Autodesk Inventor part; units mm, degrees
ref_plane "YZ Plane" through (0, 0, 0) normal (1, 0, 0) x (0, 1, 0)
ref_plane "XZ Plane" through (0, 0, 0) normal (0, 1, 0) x (-1, 0, 0)
ref_plane "XY Plane" through (0, 0, 0) normal (0, 0, 1) x (1, 0, 0)
sketch "Sketch1" plane through (0, 0, 0) normal (0, 0, 1) x (1, 0, 0)
  circle A0 centre (0, 0) radius 11.7
  dimension "d0" = 23.4
extrude "Extrusion1" add sketch "Sketch1" along normal blind 15
sketch "Sketch2" plane through (0, 0, 0) normal (0, 0, -1) x (-1, 0, 0)
  circle A0 centre (0, 0) radius 11.7
  line L0 (-11.7, 0) -> (-11.7, -20)
  line L1 (-11.7, -20) -> (11.7, -20)
  line L2 (11.7, -20) -> (11.7, 0)
  circle A1 centre (0, 0) radius 11.7
  line L3 (-11.7, 0) -> (11.7, 0)
  point P0 (11.7, 0)
  point P1 (-11.7, 0)
  dimension "d3" = 20
extrude "Extrusion2" add sketch "Sketch2" along normal blind 10
sketch "Sketch3" plane through (-11.7, -20, 0) normal (0, -1, 0) x (1, 0, 0)
  line L0 (-4.3, 22) -> (27.7, 22)
  line L1 (27.7, 22) -> (27.7, -10)
  line L2 (27.7, -10) -> (-4.3, -10)
  line L3 (-4.3, -10) -> (-4.3, 22)
  line L4 (23.4, -10) -> (0, -10)
  line L5 (23.4, 0) -> (0, 0)
  point P0 (11.7, 0)
  point P1 (11.7, 22)
  point P2 (11.7, 0)
  dimension "d6" = 32
  dimension "d7" = 32
extrude "Extrusion3" add sketch "Sketch3" along normal blind 10
sketch "Sketch4" plane through (-11.7, -30, 0) normal (0, -1, 0) x (1, 0, 0)
  line L0 (0.7, 17) -> (22.7, 17) construction
  line L1 (22.7, 17) -> (22.7, -5) construction
  line L2 (22.7, -5) -> (0.7, -5) construction
  line L3 (0.7, -5) -> (0.7, 17) construction
  line L4 (27.7, 22) -> (-4.3, 22) construction
  line L5 (-4.3, 22) -> (-4.3, -10) construction
  point P0 (11.7, 0)
  point P1 (11.7, 17)
  point P2 (11.7, 22)
  point P3 (0.7, 6)
  point P4 (-4.3, 6)
  dimension "d10" = 22
  dimension "d11" = 22
hole "Hole1" at (-11, -30, 17) at (11, -30, 17) at (11, -30, -5) at (-11, -30, -5) direction (0, 1, 0) diameter 5 depth 10
sketch "Sketch5" plane through (0, 0, 0) normal (0, 0, 1) x (1, 0, 0)
  line L0 (11.7, -20) -> (-11.7, -20)
  line L1 (5, -20) -> (-5, -20)
  line L2 (-5, -20) -> (-5, -11.7)
  line L3 (-5, -11.7) -> (5, -11.7)
  line L4 (5, -11.7) -> (5, -20)
  circle A0 centre (0, 0) radius 11.7
  line L5 (11.7, -20) -> (5, -20)
  line L6 (5, -20) -> (5, -14)
  line L7 (5, -14) -> (11.7, -14)
  line L8 (11.7, -14) -> (11.7, -20)
  line L9 (-5, -20) -> (-11.7, -20)
  line L10 (-11.7, -20) -> (-11.7, -14)
  line L11 (-11.7, -14) -> (-5, -14)
  line L12 (-5, -14) -> (-5, -20)
  line L13 (-11.7, -20) -> (-11.7, 0)
  line L14 (11.7, 0) -> (11.7, -20)
  point P0 (0, -11.7)
  dimension "d19" = 10
  dimension "d20" = 6
extrude "Extrusion4" cut sketch "Sketch5" against normal through all contours L0 L4 L7 L8 | L0 L10 L11 L2
chamfer "Chamfer1" distance 1 distance2 3 1 edges at (-11.7, 0, 15) measured on face at (-1.2696, -2.7132, 15)
equation "\"d7\" = d6"
equation "\"d11\" = d10"
properties part number "0008-30-004"
Source: CAD feature listing. Evaluate the final solid. Frame: model axes, mm. A direction names the side the tool comes from. Give positions to 0.01 mm unless a question says otherwise; leave off trailing zeros. Order: outer loops, then holes, each group sorted by start corner. A loop starts at its lowest first (then second) coordinate and runs counter-clockwise, first axis right, second up. Notation, with made-up numbers: (37.25, 59) -> (42.25, 59) arc R29 ccw to (42.25, 96) -> close; hole circle Ø1 at (67.25, 19). An arc over 180 degrees is marked (long way). Write item = value, one per line.
Item 1: Mould query, pull axis Y, two halves, no side actions, for faces 5 (the face through (5.4, 10.38, 3.29)), 6 (the face through (11.7, -7, -5)), 7 (the face through (0, -30, 6)). Classes: +Y half, -Y half, draft (parallel to the pull), parting line (faces both ways), or undercut.
Check result:
face_5 = undercut
face_6 = draft
face_7 = -Y half
Item 2: Section query A-A (z = -5). Output: boundary loops of the cut face in (x, y), then the cut area to 3 significant figures.
Check result:
outline = (-16, -30) -> (-13.5, -30) -> (-13.5, -20) -> (-16, -20) -> close; (-11.7, -14) -> (-5, -14) -> (-5, -20) -> (-8.5, -20) -> (-8.5, -30) -> (8.5, -30) -> (8.5, -20) -> (5, -20) -> (5, -14) -> (11.7, -14) -> (11.7, 0) arc R11.7 ccw to (-11.7, 0) -> close; (13.5, -30) -> (16, -30) -> (16, -20) -> (13.5, -20) -> close
area = 823 mm²
Item 3: Section query D-D (z = -1.5). Output: boundary loops of the cut face in (x, y), then the cut area to 3 significant figures.
Check result:
outline = (-16, -30) -> (16, -30) -> (16, -20) -> (5, -20) -> (5, -14) -> (11.7, -14) -> (11.7, 0) arc R11.7 ccw to (-11.7, 0) -> (-11.7, -14) -> (-5, -14) -> (-5, -20) -> (-16, -20) -> close
area = 923 mm²
Item 4: Set-up query: faces 1 (the face through (0, 0, 15)), 2 (the face through (0, -14, 0)), 3 (the face through (-8, -14, -5)), 4 (the face through (-8.78, -24.93, -6.15)). Return all of +Z, -Z, +X, -X, +Y, -Y with unobstructed straight access to the full face (end or side cutting, diameter ignored); none if empty.
Check result:
face_1 = +Z, +X, -X, +Y
face_2 = +Z
face_3 = +Z, -Z, -X
face_4 = -Y
Item 5: Section query C-C (z = 9). Output: boundary loops of the cut face in (x, y), then the cut area to 3 significant figures.
Check result:
outline = (-16, -30) -> (16, -30) -> (16, -20) -> (-16, -20) -> close; circle Ø23.4 at (0, 0)
area = 750 mm²
Item 6: Contact query for flat-ended pins moving along their axis: pin 1 (6 mm diameter, centred on x = 9, y = 6.5, fed in from +Z); pin 2 (8 mm diameter, centred on x = -11, z = 3.5, fed in from +Y); pin 3 (12 mm diameter, centred on y = 1, z = 3, fed in from -X). Output: stop coordinate, or through.
Check result:
pin_1 = 15
pin_2 = 9.37
pin_3 = -11.7
Item 7: Section query B-B (x = 0). Output: boundary loops of the cut face in (y, z).
Check result:
outline = (-30, -10) -> (11.7, -10) -> (11.7, 12) -> (10.7, 15) -> (-10.7, 15) -> (-11.7, 12) -> (-11.7, 0) -> (-20, 0) -> (-20, 22) -> (-30, 22) -> close
Item 8: Ray query, probe 1 along X at (y, z) = (-22.25, -5); probe 2 along Z at (x, y) = (-12.5, -28); probe 3 along Y at (x, z) = (-11.5, 14.5). Return the intervals inside material, ascending.
Check result:
probe_1 = -16 to -13.5, -8.5 to 8.5, 13.5 to 16
probe_2 = -10 to -7, -3 to 15, 19 to 22
probe_3 = -30 to -20
